The model under review builds one solid part; all positions refer to its coordinate system, in mm. A direction names the side the tool comes from. Round coordinates to 2 decimals unless told otherwise and drop trailing zeros. Loops run counter-clockwise (first coordinate to the right, second up) from the corner with the lowest first, then second, coordinate; pieces in that order, holes last. Notation, with made-up numbers: (-23, 67.5) -> (33, 67.5) arc R31 ccw to (33, 95.5) -> close; hole circle Ø7 at (25.5, 20.25). An arc over 180 degrees is marked (long way). Use CSV: the item, a comma, the result in double quotes. Start each with the question number.
```python
from build123d import *

# Parameters (mm, degrees)
SKETCH1_W               = 27.6225
SKETCH1_H               = 11.7348
BOSS_EXTRUDE1_DEPTH     = 7.112
CUT_EXTRUDE1_DEPTH      = 46.755458387
CUT_EXTRUDE1_DEPTH_BACK = 46.755458387
SKETCH3_W               = 5.08
SKETCH3_H               = 4.826
CUT_EXTRUDE2_DEPTH      = 10.5918
CUT_EXTRUDE3_REACH      = 56.598
SKETCH4_W               = 21.32965
SKETCH4_H               = 7.8994


with BuildPart() as part:
    # Sketch1 → Boss-Extrude1 (new body)
    with BuildSketch(Plane(origin=(0, 0, 0), x_dir=(1, 0, 0), z_dir=(0, 1, 0))):
        with Locations((-29.838216172, 26.150202934)):
            Rectangle(SKETCH1_W, SKETCH1_H)
    extrude(amount=BOSS_EXTRUDE1_DEPTH)

    # Sketch2 → Cut-Extrude1 (cut, two sides: drawn at the far end of the back side and taken through both)
    with BuildSketch(Plane.XY.offset(-20.282802934).offset(-CUT_EXTRUDE1_DEPTH_BACK)):
        Polygon((-36.283466172, 73.446090762), (-36.283466172, 7.112), (-36.283466172, 5.5118), (-29.990616172, 5.5118), (-29.990616172, 6.8834), (-22.319816172, 6.8834), (-22.319816172, 5.5118), (-16.026966172, 5.5118), (50.307124589, 5.5118), (132.196959284, 109.890444188), (45.606368522, 177.82473495), align=None)
    extrude(amount=CUT_EXTRUDE1_DEPTH + CUT_EXTRUDE1_DEPTH_BACK, mode=Mode.SUBTRACT)

    # Sketch3 → Cut-Extrude2 (cut)
    with BuildSketch(Plane.XY.offset(-20.282802934)):
        with Locations((-39.966466172, 3.556)):
            Rectangle(SKETCH3_W, SKETCH3_H)
        Polygon((-35.140466172, 4.3688), (-35.140466172, 1.143), (-17.169966172, 1.143), (-17.169966172, 4.3688), (-23.462816172, 4.3688), (-23.462816172, 5.7404), (-28.847616172, 5.7404), (-28.847616172, 4.3688), align=None)
    extrude(amount=-CUT_EXTRUDE2_DEPTH, mode=Mode.SUBTRACT)

    # Cut-Extrude3: up to this face of the body (flat: up to its plane)
    cut_extrude3_end = Plane(part.part.faces().sort_by_distance((-33.137041172, 5.5118, -26.150202934))[0])
    # Sketch4 → Cut-Extrude3 (cut, up to the picked face)
    with BuildSketch(Plane(origin=(0, 7.112, 0), x_dir=(1, 0, 0), z_dir=(0, 1, 0)), mode=Mode.PRIVATE) as cut_extrude3_sk1:
        with Locations((-32.984641172, 28.067902934)):
            Rectangle(SKETCH4_W, SKETCH4_H)
    cut_extrude3_tool1 = split(extrude(cut_extrude3_sk1.sketch, amount=-CUT_EXTRUDE3_REACH, mode=Mode.PRIVATE), bisect_by=cut_extrude3_end, keep=Keep.BOTH, mode=Mode.PRIVATE)
    add(cut_extrude3_tool1.solids().sort_by(Axis((-32.984641, 7.112, -28.067903), (0, -1, 0)))[0], mode=Mode.SUBTRACT)


solid = part.part
```
1. The part is to be moulded in two halves that separate along X. For faces 1 (the face through (-22.32, 6, -22)), 2 (the face through (-26, 3, -30.875)), 3 (the face through (-40, 6.5, -24.118)), say which applies: pulls with the +X half, pulls with the -X half, needs draft (parallel to the pull), parting line crosses it, or undercut.
2. Take a section at C-C, the plane y = 4. Give the boundary of the cut face in (x, z).
3. For faces 4 (the face through (-26, 6.883, -22)), 5 (the face through (-28.848, 5, -26)), 6 (the face through (-40, 3, -30.875)), list the 3-axis set-ups (+Z, -Z, +X, -X, +Y, -Y) from which the entire face can be reached by the end or side of a thin tool; tool diameter is ignored.
4. Take a section at D-D, the plane x = -21.5. Give the boundary of the cut face in (y, z), then the cut area to 3 significant figures.
5. Take a section at A-A, the plane x = -28. Give the boundary of the cut face in (y, z).
6. Take a section at B-B, the plane z = -21. Give the boundary of the cut face in (x, y), then the cut area to 3 significant figures.
7. For line 1 along X through (y, z) = (5, -30.25); line 2 along X through (y, z) = (3, -29); line 3 along Y through (x, z) = (-19.75, -27), list the stretches that pass through material, from the lowest coordinate up. Write a range as from..to.
8. Clearance check with flat-ended pins moving along their axes: P1, Ø3.5, axis at x = -40, y = 3, coming from the +Z side; P2, Ø0.7, axis at y = 6, z = -22.5, coming from the +X side; P3, Ø1.3, axis at x = -40.5, y = 6.5, coming from the -Z side. State where each tip first meets the part, or that it passes through.
Results:
1,face 1,"pulls with the +X half"
1,face 2,"undercut"
1,face 3,"needs draft"
2,outline,"(-43.65, -32.02) -> (-16.03, -32.02) -> (-16.03, -20.28) -> (-17.17, -20.28) -> (-17.17, -30.87) -> (-35.14, -30.87) -> (-35.14, -20.28) -> (-37.43, -20.28) -> (-37.43, -30.87) -> (-42.51, -30.87) -> (-42.51, -20.28) -> (-43.65, -20.28) -> close"
3,face 4,"+Z, -Z, +X, +Y"
3,face 5,"+Z"
3,face 6,"+Z, +Y"
4,outline,"(0, -32.02) -> (5.51, -32.02) -> (5.51, -20.28) -> (4.37, -20.28) -> (4.37, -30.87) -> (1.14, -30.87) -> (1.14, -20.28) -> (0, -20.28) -> close"
4,area,"30.5 mm²"
5,outline,"(0, -32.02) -> (5.51, -32.02) -> (5.51, -30.87) -> (1.14, -30.87) -> (1.14, -20.28) -> (0, -20.28) -> close; (5.74, -24.12) -> (6.88, -24.12) -> (6.88, -20.28) -> (5.74, -20.28) -> close"
6,outline,"(-43.65, 0) -> (-16.03, 0) -> (-16.03, 5.51) -> (-22.32, 5.51) -> (-22.32, 6.88) -> (-29.99, 6.88) -> (-29.99, 5.51) -> (-36.28, 5.51) -> (-36.28, 7.11) -> (-43.65, 7.11) -> close; hole (-42.51, 1.14) -> (-37.43, 1.14) -> (-37.43, 5.97) -> (-42.51, 5.97) -> close; hole (-35.14, 1.14) -> (-17.17, 1.14) -> (-17.17, 4.37) -> (-23.46, 4.37) -> (-23.46, 5.74) -> (-28.85, 5.74) -> (-28.85, 4.37) -> (-35.14, 4.37) -> close"
6,area,"84.7 mm²"
7,line 1,"-43.65..-42.51, -37.43..-28.85, -23.46..-16.03"
7,line 2,"-43.65..-42.51, -37.43..-35.14, -17.17..-16.03"
7,line 3,"0..1.14, 4.37..5.51"
8,P1,"z = -30.87"
8,P2,"x = -22.32"
8,P3,"z = -24.12"
